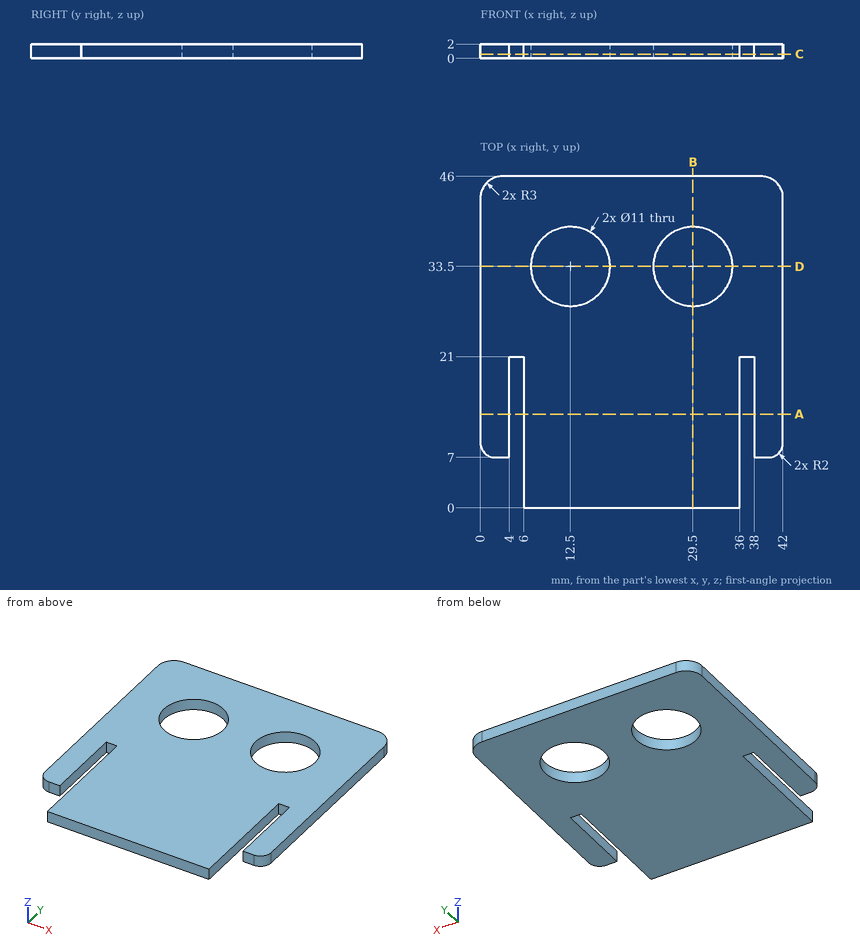
Drawing for the job (mm, zero at the part's lowest x, y, z). Give positions to 0.01 mm unless a question says otherwise; leave off trailing zeros. Order: outer loops, then holes, each group sorted by start corner. A loop starts at its lowest first (then second) coordinate and runs counter-clockwise, first axis right, second up. Notation, with made-up numbers: M -20,88.5 L 29,88.5 A14 cw 29,107.5 Z; hole C 8,-18 d10. An arc over 180 degrees is marked long. Write item = value, one per line. Start each with the question number.
(1) Pin check, flat tips, straight feed: pin 1 Ø1 at (x, y) = (9.5, 30.5) entering from -Z; pin 2 Ø0.6 at (x, z) = (4.5, 1) entering from -Y; pin 3 Ø1 at (x, z) = (3, 1) entering from -Y. Stop position of each tip, or through.
(2) Slice it at C-C on z = 0.6. Write the cut outline in (x, y).
(3) Slice it at A-A on y = 13. Write the cut outline in (x, z), plus the area to 3 significant figures.
(4) Probe L1, parallel to X at y = 13.5, z = 0.1; L2, parallel to Y at x = 12.5, z = 0.95; L3, parallel to X at y = 37, z = 0.9. List the from-to ranges inside material, lowest first. Write a range as [from, to].
(5) Slice it at B-B on x = 29.5. Write the cut outline in (y, z).
(6) Slice it at D-D on y = 33.5. Write the cut outline in (x, z).
Responses:
q1.pin_1 = through
q1.pin_2 = 21
q1.pin_3 = 7
q2.outline = M 0,9 A2 ccw 2,7 L 4,7 L 4,21 L 6,21 L 6,0 L 36,0 L 36,21 L 38,21 L 38,7 L 40,7 A2 ccw 42,9 L 42,43 A3 ccw 39,46 L 3,46 A3 ccw 0,43 Z; hole C 12.5,33.5 d11; hole C 29.5,33.5 d11
q3.outline = M 0,0 L 4,0 L 4,2 L 0,2 Z; M 6,0 L 36,0 L 36,2 L 6,2 Z; M 38,0 L 42,0 L 42,2 L 38,2 Z
q3.area = 76.0 mm2
q4.L1 = [0, 4], [6, 36], [38, 42]
q4.L2 = [0, 28], [39, 46]
q4.L3 = [0, 8.26], [16.74, 25.26], [33.74, 42]
q5.outline = M 0,0 L 28,0 L 28,2 L 0,2 Z; M 39,0 L 46,0 L 46,2 L 39,2 Z
q6.outline = M 0,0 L 7,0 L 7,2 L 0,2 Z; M 18,0 L 24,0 L 24,2 L 18,2 Z; M 35,0 L 42,0 L 42,2 L 35,2 Z
